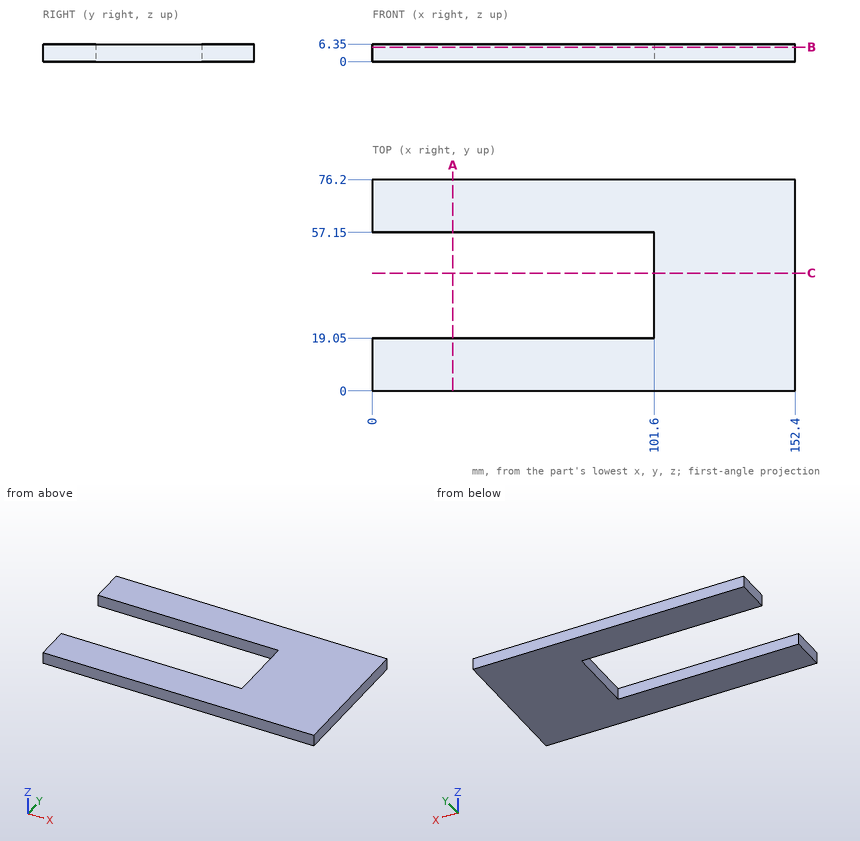
Can you work these out from the drawing? Everything is in mm from the part's minimum corner. Coordinates: 2 decimals unless noted, no trailing zeros. Write each loop counter-clockwise with the first axis right and the second up, starting at its lowest first coordinate (ties: lowest second). Pieces come first, ordered by that corner, then holes. Notation, with made-up numbers: (-18, 47.25) - (9, 47.25) arc R29 cw to (9, 84.25) - close; hole circle Ø2 at (81, -21.5). An arc over 180 degrees is marked (long way). One line per item, written item: value.
1) Suppose I cut it at B-B on z = 5.25. Write out the boundary of the cut face in (x, y), and give its area (3 significant figures).
Model answer:
outline: (0, 0) - (152.4, 0) - (152.4, 76.2) - (0, 76.2) - (0, 57.15) - (101.6, 57.15) - (101.6, 19.05) - (0, 19.05) - close
area: 7,740 mm²
2) I need wall thicknesses on line 1 along Y through (x, z) = (49, 4); line 2 along X through (y, z) = (44.5, 6). Which ranges of each line are inside material? Lowest first, please.
Model answer:
line 1: y = 0 to 19.05, 57.15 to 76.2
line 2: x = 101.6 to 152.4
3) Suppose I cut it at C-C on y = 42.5. Write out the boundary of the cut face in (x, z), and give its area (3 significant figures).
Model answer:
outline: (101.6, 0) - (152.4, 0) - (152.4, 6.35) - (101.6, 6.35) - close
area: 323 mm²
4) Suppose I cut it at A-A on x = 29. Write out the boundary of the cut face in (y, z), and give its area (3 significant figures).
Model answer:
outline: (0, 0) - (19.05, 0) - (19.05, 6.35) - (0, 6.35) - close; (57.15, 0) - (76.2, 0) - (76.2, 6.35) - (57.15, 6.35) - close
area: 242 mm²
5) I'm going to push a flat-ended pin straight in: P1, Ø3, axis at y = 38, z = 2.5, coming from the -X side. Where does the tip first touch, or does it pass through?
Model answer:
P1: stops at x = 101.6
